Part model, mm, in its own coordinate system. Face numbers are marked on the shaded views. A direction names the side the tool comes from. Give positions to 0.01 mm unless a question says otherwise; leave off trailing zeros. Order: outer loops, then holes, each group sorted by start corner. A loop starts at its lowest first (then second) coordinate and runs counter-clockwise, first axis right, second up. Notation, with made-up numbers: (6, -7) -> (56, -7) arc R23 ccw to (56, 5) -> close; hole circle Ø9 at (-27, 78). An arc over 180 degrees is marked (long way). Write item = value, one per line. Start each with the question number.
(1) Probe line 1 along Z through (x, y) = (0, -3); line 2 along X through (y, z) = (2.5, 0.5); line 3 along Z through (x, y) = (-34.5, -1.75). List the from-to ranges inside material, lowest first. Write a range as from..to.
(2) Saw through at D-D, the plane x = -32. List the corners of the cut face in (y, z).
(3) Which spindle directions (+Z, -Z, +X, -X, +Y, -Y) get a long thin tool onto all of the face, cutting with end or side? Do the marked faces 4 and 5. Say none if no direction does.
(4) Two-plate mould, pull along X, no slides. Class the marked faces 1, 2 and 3: pulls with the +X half, pulls with the -X half, needs draft (parallel to the pull), parting line crosses it, or undercut.
(5) Flat gauge pin, fed straight in: pin 1 (2 mm diameter, centred on x = -1.5, z = -1.5, fed in from -Y). Where does the tip first touch, or does it go through?
(6) Saw through at B-B, the plane y = 2.75. List the corners of the cut face in (x, z), then the cut area to 3 significant figures.
(7) Saw through at C-C, the plane z = -3.5. List the corners of the cut face in (x, y), then the cut area to 3 significant figures.
(8) Saw through at A-A, the plane x = 0. List the corners of the cut face in (y, z), then the cut area to 3 significant figures.
from build123d import *

# Parameters (mm, degrees)
SKETCH_1_R      = 4
EXTRUDE_1_DEPTH = 5


with BuildPart() as part:
    # 草圖1 → 填料-伸長1 (new body, symmetric)
    with BuildSketch(Plane(origin=(0, 0, 0), x_dir=(1, 0, 0), z_dir=(0, 1, 0))):
        Polygon((-40, -5), (-40, 0), (-30, 0), (-30, -5), (6, -5), (6, 5), (-42, 5), (-42, -5), align=None)
        Circle(SKETCH_1_R, mode=Mode.SUBTRACT)
    extrude(amount=EXTRUDE_1_DEPTH, both=True)


solid = part.part
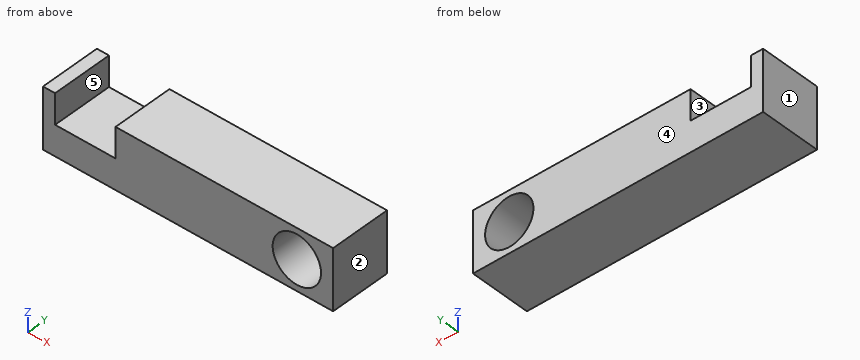
Results list:
q1.line_1 = -5..-4, 4..5
q1.line_2 = -42..-40, -30..-3.97, 3.97..6
q1.line_3 = -5..0
q2.outline = (-5, -5) -> (5, -5) -> (5, 0) -> (-5, 0) -> close
q3.face_4 = +Z, -Z, +X, -X, +Y
q3.face_5 = +Z, +Y, -Y
q4.face_1 = pulls with the -X half
q4.face_2 = pulls with the +X half
q4.face_3 = undercut
q5.pin_1 = through
q6.outline = (-42, -5) -> (6, -5) -> (6, 5) -> (-30, 5) -> (-30, 0) -> (-40, 0) -> (-40, 5) -> (-42, 5) -> close; hole circle Ø8 at (0, 0)
q6.area = 380 mm^2
q7.outline = (-42, -5) -> (-1.94, -5) -> (-1.94, 5) -> (-42, 5) -> close; (1.94, -5) -> (6, -5) -> (6, 5) -> (1.94, 5) -> close
q7.area = 441 mm^2
q8.outline = (-5, -5) -> (5, -5) -> (5, -4) -> (-5, -4) -> close; (-5, 4) -> (5, 4) -> (5, 5) -> (-5, 5) -> close
q8.area = 20.0 mm^2
